Part model, mm, in its own coordinate system. Coordinates: 2 decimals unless noted, no trailing zeros. Write each loop counter-clockwise with the first axis right and the second up, starting at its lowest first coordinate (ties: lowest second). Pieces come first, ordered by that corner, then holes. Notation, with made-up numbers: M 41,-18.75 L 53,-18.75 A25 ccw 53,3.25 Z; hole C -32.75,-15.5 d8. An arc over 180 degrees is marked long. Use a Markdown table: item, result. Add a question column.
Q1. Pin check, flat tips, straight feed: pin 1 Ø5 at (x, z) = (38.5, -4) entering from -Y; pin 2 Ø1 at (x, z) = (61.5, 2) entering from -Y; pin 3 Ø3 at (x, y) = (44.5, 12) entering from +Z. Stop position of each tip, or through.
Q2. Slice it at D-D on z = -3. Write the cut outline in (x, y).
Q3. Slice it at C-C on z = -15. Write the cut outline in (x, y).
Q4. Slice it at A-A on y = 12.75. Write the cut outline in (x, z), then the cut area to 3 significant figures.
Q5. Slice it at B-B on x = 61.5. Write the cut outline in (y, z).
Q6. Wall check: L1, parallel to Z at x = 65.5, y = 9.25; L2, parallel to Z at x = 15.5, y = -10.5; L3, parallel to Y at x = 18, z = 4.5. Give the ranges that are in metal, low to high. Write a range as from..to.
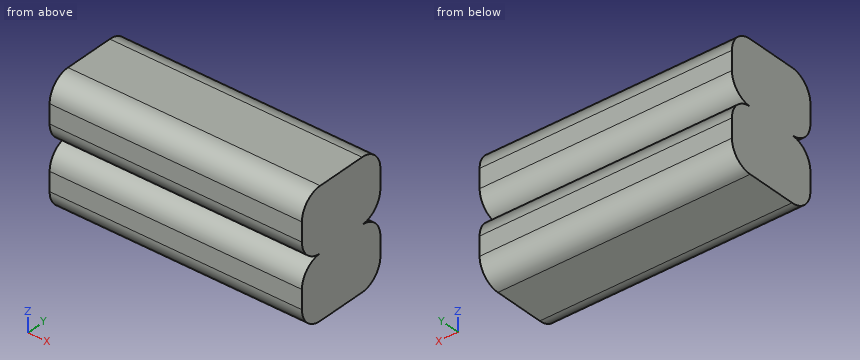
from build123d import *

# Parameters (mm, degrees)
EXTRUDE_1_DEPTH = 80
FILLET_1_R      = 7
FILLET_2_R      = 7
FILLET_3_R      = 7
FILLET_4_R      = 7


with BuildPart() as part:
    # 草图1 → 凸台-拉伸1 (new body)
    with BuildSketch(Plane(origin=(0, 0, 0), x_dir=(0, 0, -1), z_dir=(1, 0, 0))):
        with BuildLine():
            Line((20, -15), (7, -15))
            ThreePointArc((7, -15), (2.050252532, -12.949747468), (0, -8))
            ThreePointArc((0, -8), (-2.050252532, -12.949747468), (-7, -15))
            Line((-7, -15), (-20, -15))
            Line((-20, -15), (-20, 15))
            Line((-20, 15), (-7, 15))
            ThreePointArc((-7, 15), (-2.050252532, 12.949747468), (0, 8))
            ThreePointArc((0, 8), (2.050252532, 12.949747468), (7, 15))
            Line((7, 15), (20, 15))
            Line((20, 15), (20, -15))
        make_face()
    extrude(amount=EXTRUDE_1_DEPTH)

    # 圆角1
    fillet_1_edges = [part.edges().sort_by_distance(p)[0] for p in [
        (40, 15, -20),
    ]]
    fillet(fillet_1_edges, radius=FILLET_1_R)

    # 圆角2
    fillet_2_edges = [part.edges().sort_by_distance(p)[0] for p in [
        (40, 15, 20),
    ]]
    fillet(fillet_2_edges, radius=FILLET_2_R)

    # 圆角3
    fillet_3_edges = [part.edges().sort_by_distance(p)[0] for p in [
        (40, -15, -20),
    ]]
    fillet(fillet_3_edges, radius=FILLET_3_R)

    # 圆角4
    fillet_4_edges = [part.edges().sort_by_distance(p)[0] for p in [
        (40, -15, 20),
    ]]
    fillet(fillet_4_edges, radius=FILLET_4_R)


solid = part.part
Recorded:
| question | item | result |
|---|---|---|
| 1 | pin 1 | y = -14.98 |
| 1 | pin 2 | y = -13.36 |
| 1 | pin 3 | z = 19.54 |
| 2 | outline | M 0,-13.74 L 80,-13.74 L 80,13.74 L 0,13.74 Z |
| 3 | outline | M 0,-14.71 L 80,-14.71 L 80,14.71 L 0,14.71 Z |
| 4 | outline | M 0,-18.14 L 80,-18.14 L 80,-1.86 L 0,-1.86 Z; M 0,1.86 L 80,1.86 L 80,18.14 L 0,18.14 Z |
| 4 | area | 2,610 mm² |
| 5 | outline | M -15,-13 A7 ccw -8,-20 L 8,-20 A7 ccw 15,-13 L 15,-7 A7 ccw 8,0 A7 ccw 15,7 L 15,13 A7 ccw 8,20 L -8,20 A7 ccw -15,13 L -15,7 A7 ccw -8,0 A7 ccw -15,-7 Z |
| 6 | L1 | -19.89..-0.11, 0.11..19.89 |
| 6 | L2 | -19.54..-0.46, 0.46..19.54 |
| 6 | L3 | -14.54..14.54 |
